Geometry: final body of the model. Coordinates: model frame, mm. A direction names the side the tool comes from. Give positions to 0.01 mm unless a question says otherwise; leave off trailing zeros. Order: outer loops, then holes, each group sorted by start corner. A loop starts at its lowest first (then second) coordinate and runs counter-clockwise, first axis right, second up. Notation, with made-up numbers: (56.5, 60.5) -> (73.5, 60.5) arc R19 cw to (73.5, 67.5) -> close; hole circle Ø9 at (83.5, 11). An arc over 180 degrees is marked (long way). Write item = value, one per line.
Autodesk Inventor part; units mm, degrees
ref_plane "YZ Plane" through (0, 0, 0) normal (1, 0, 0) x (0, 1, 0)
ref_plane "XZ Plane" through (0, 0, 0) normal (0, 1, 0) x (-1, 0, 0)
ref_plane "XY Plane" through (0, 0, 0) normal (0, 0, 1) x (1, 0, 0)
sketch "Sketch1" plane through (0, 0, 0) normal (0, 1, 0) x (-1, 0, 0)
  line L0 (-34.6421, 35) -> (34.6421, 35)
  line L1 (34.6421, 35) -> (34.6421, -35)
  line L2 (34.6421, -35) -> (-34.6421, -35)
  line L3 (-34.6421, -35) -> (-34.6421, 35)
  line L4 (-34.6421, 35) -> (34.6421, -35) construction
  line L5 (34.6421, 35) -> (-34.6421, -35) construction
  point P0 (0, 0)
  dimension "d0" = 70
extrude "Extrusion1" add sketch "Sketch1" along normal blind 5
fillet "Fillet1" radius 2 4 edges at (-34.6421, 2.5, -35) (-34.6421, 2.5, 35) (34.6421, 2.5, 35) (34.6421, 2.5, -35)
sketch "Sketch2" plane through (0, 0, 0) normal (0, -1, 0) x (1, 0, 0)
  line L0 (36.6421, 1) -> (34.6421, 1)
  line L1 (34.6421, 1) -> (34.6421, -1)
  line L2 (34.6421, -1) -> (36.6421, -1)
  line L3 (36.6421, -1) -> (36.6421, 1)
  line L4 (36.6421, 1) -> (34.6421, -1) construction
  line L5 (34.6421, 1) -> (36.6421, -1) construction
  arc A0 (38.6405, 1.5334) -> (38.6405, -1.5334) centre (38.2296, 0) ccw
  line L6 (34.6421, 33) -> (34.6421, -33)
  line L7 (35.6421, 0) -> (34.6421, 0) construction
  arc A1 (38.9511, 2.6925) -> (38.9511, -2.6925) centre (38.2296, 0) ccw
  line L8 (38.9511, 2.6925) -> (38.6405, 1.5334)
  line L9 (38.6405, -1.5334) -> (38.9511, -2.6925)
  point P0 (0, 0)
  point P1 (36.6421, 0)
  point P2 (35.6277, 1)
  point P3 (35.6277, -1)
  dimension "d4" = 150
  dimension "d5" = 1.5875
  dimension "d6" = 2
  dimension "d8" = 150
  dimension "d9" = 1.2
extrude "Extrusion2" add sketch "Sketch2" against normal up to surface (5 mm away)
sketch "Sketch3" plane through (0, 5, 0) normal (0, 1, 0) x (1, 0, 0)
  circle A0 centre (-29.6421, -30) radius 3.25
  line L0 (-34.6421, 33) -> (-34.6421, -33)
  line L1 (-32.6421, -35) -> (32.6421, -35)
  circle A1 centre (-29.6421, 30) radius 3.25
  circle A2 centre (30.3579, -30) radius 3.25
  circle A3 centre (30.3579, 30) radius 3.25
  point P0 (0, 0)
  dimension "d12" = 6.5
  dimension "d15" = 60
  dimension "d18" = 60
  dimension "d21" = 5
  dimension "d22" = 5
extrude "Extrusion3" cut sketch "Sketch3" against normal up to surface (5 mm away)
sketch "Sketch4" plane through (0, 5, 0) normal (0, 1, 0) x (1, 0, 0)
  arc A0 (0, 8.25) -> (0, -8.25) centre (0, 0) ccw
  arc A1 (0, 11.25) -> (0, -11.25) centre (0, 0) ccw
  line L0 (0, 8.25) -> (0, 11.25)
  line L1 (0, -8.25) -> (0, -11.25)
  line L2 (0, 0) -> (0, 8.25) construction
  dimension "d25" = 8.25
  dimension "d26" = 3
  dimension "d27" = 180
revolve "Revolution1" add sketch "Sketch4" angle 90 about axis through (0, 5, 8.25) along (0, 0, -1)
sketch "Sketch5" plane through (0, 5, 0) normal (0, 1, 0) x (1, 0, 0)
  line L0 (0, 8.25) -> (0, -8.25)
  circle A0 centre (0, 0) radius 8.25
extrude "Extrusion4" cut sketch "Sketch5" against normal up to surface (5 mm away)
sketch "Sketch6" plane through (0, 5, 0) normal (0, 1, 0) x (1, 0, 0)
  circle A0 centre (0, 0) radius 2.5
  dimension "d31" = 5
extrude "Extrusion5" cut sketch "Sketch6" along normal through all
equation "\"d0\" = cradle_width"
equation "\"d1\" = cradle_slider_thickness"
equation "\"d5\" = 0.5 * tubing_diameter"
equation "\"d10\" = cradle_slider_thickness"
equation "\"d12\" = rod_diameter + rod_free_tolerance"
equation "\"d15\" = rod_dist"
equation "\"d18\" = rod_dist"
equation "\"d21\" = -0.5 * rod_dist + 0.5 * cradle_width"
equation "\"d22\" = -0.5 * rod_dist + 0.5 * cradle_width"
equation "\"d25\" = 0.5 * tube_diameter"
equation "\"d31\" = tube_tip_diameter"
equation "\"cradle_width\" = 70"
equation "\"cradle_slider_thickness\" = 5"
equation "\"tubing_diameter\" = 3.175"
equation "\"rod_diameter\" = 6"
equation "\"rod_free_tolerance\" = 0.5"
equation "\"tube_diameter\" = 16.5"
equation "\"tube_tip_diameter\" = 5"
equation "\"rod_dist\" = 60"
properties part number "cradle_slider"
1) Section query A-A (z = 30). Output: boundary loops of the cut face in (x, y).
Check sheet entries:
outline = (-34.64, 0) -> (-32.89, 0) -> (-32.89, 5) -> (-34.64, 5) -> close; (-26.39, 0) -> (27.11, 0) -> (27.11, 5) -> (-26.39, 5) -> close; (33.61, 0) -> (34.64, 0) -> (34.64, 5) -> (33.61, 5) -> close
2) Reachability of faces 4 (the face through (0, 11, -7)), 5 (the face through (36.94, 2.46, -2.47)), 6 (the face through (7.62, 2.54, 3.16)) from +Z, -Z, +X, -X, +Y, -Y: full face, straight path, thin tool, end or side. Return the list, or none.
Check sheet entries:
face_4 = +Z, -Z, +X, +Y
face_5 = -Z, +Y, -Y
face_6 = -Y
3) Line query: line 1 (X direction, y = 3.9, z = 30); line 2 (Z direction, x = 30, y = 3); line 3 (Z direction, x = 0, y = 3.7). Output: solid intervals per line, ascending. Write a range as from..to.
Check sheet entries:
line_1 = -34.64..-32.89, -26.39..27.11, 33.61..34.64
line_2 = -35..-33.23, -26.77..26.77, 33.23..35
line_3 = -35..-8.25, 8.25..35
4) Section query B-B (z = 0). Output: boundary loops of the cut face in (x, y), plus the area to 3 significant figures.
Check sheet entries:
outline = (-34.64, 0) -> (-8.25, 0) -> (-8.25, 5) arc R8.25 cw to (-2.5, 12.86) -> (-2.5, 15.97) arc R11.25 ccw to (-11.25, 5) -> (-34.64, 5) -> close; (8.25, 0) -> (36.64, 0) -> (36.64, 5) -> (8.25, 5) -> close
area = 312 mm²
5) First-contact query: P1, Ø5, axis at x = -29.64, z = -30, coming from the +Y side; P2, Ø0.8, axis at x = 35.5, y = 2.5, coming from the +Z side; P3, Ø8.5, axis at x = 30.36, z = -30, coming from the +Y side; P4, Ø2.5, axis at y = 1.5, z = 17, coming from the +X side. Flat tips, straight axial feed; report the tip coordinate or a pass-through.
Check sheet entries:
P1 = through
P2 = 1.53
P3 = 5
P4 = 34.64
6) Section query C-C (x = -4). Output: boundary loops of the cut face in (y, z), plus the area to 3 significant figures.
Check sheet entries:
outline = (0, -35) -> (5, -35) -> (5, -10.51) arc R10.51 ccw to (5, 10.51) -> (5, 35) -> (0, 35) -> (0, 7.22) -> (5, 7.22) arc R7.22 cw to (5, -7.22) -> (0, -7.22) -> close
area = 370 mm²
7) Mould query, pull axis X, two halves, no side actions, for faces 1 (the face through (-34.642, 2, 0)), 2 (the face through (-2.5, 14.4, 0.1)), 3 (the face through (31.86, 2.54, 32.88)). Classes: +X half, -X half, draft (parallel to the pull), parting line (faces both ways), or undercut.
Check sheet entries:
face_1 = -X half
face_2 = +X half
face_3 = undercut
8) Section query D-D (y = 14.5). Output: boundary loops of the cut face in (x, z).
Check sheet entries:
outline = (0, -6.03) -> (0, -2.5) arc R2.5 cw to (0, 2.5) -> (0, 6.03) arc R6.03 ccw to start
